Model file for the job. Use its own axes, mm. A direction names the side the tool comes from. Round coordinates to 2 decimals unless told otherwise and drop trailing zeros. Loops run counter-clockwise (first coordinate to the right, second up) from the corner with the lowest first, then second, coordinate; pieces in that order, holes last. Notation, with made-up numbers: (1, -32) -> (31, -32) arc R31 ccw to (31, 7) -> close; hole circle Ø1 at (75, -40). An arc over 180 degrees is marked (long way). Use a Markdown table: item, result. Add a question column.
```python
from build123d import *

# Parameters (mm, degrees)
EXTRUDE_1_DEPTH     = 4
CUT_EXTRUDE_1_DEPTH = 1.5
CUT_EXTRUDE_2_DEPTH = 7.5


with BuildPart() as part:
    # Эскиз1 → Бобышка-Вытянуть1 (new body, symmetric)
    with BuildSketch(Plane.XY):
        Polygon((4, 0), (-4, 0), (-4, -1.5), (-9.75, -1.5), (-9.75, -8), (9.75, -8), (9.75, -1.5), (4, -1.5), align=None)
    extrude(amount=EXTRUDE_1_DEPTH, both=True)

    # Эскиз3 → Отверстие обработанное метчиком M62 (revolve, cut)
    with BuildSketch(Plane(origin=(0, 0, 0), x_dir=(0, 0, 1), z_dir=(1, 0, 0))):
        Polygon((0, 0), (0, 8), (3.5, 8), (2.5, 7), (2.5, 1), (3.5, 0), align=None)
    revolve(axis=Axis((0, 6.35, 0), (0, -1, 0)), mode=Mode.SUBTRACT)

    # Эскиз4 → Вырез-Вытянуть1 (cut)
    with BuildSketch(Plane(origin=(0, 0, 0), x_dir=(1, 0, 0), z_dir=(0, 1, 0))):
        with BuildLine():
            Line((-4, 4), (-4, 0))
            ThreePointArc((-4, 0), (-2.828427125, 2.828427125), (0, 4))
            Line((0, 4), (-4, 4))
        make_face()
        with BuildLine():
            Line((0, -4), (4, -4))
            Line((4, -4), (4, 0))
            ThreePointArc((4, 0), (2.828427125, -2.828427125), (0, -4))
        make_face()
    extrude(amount=-CUT_EXTRUDE_1_DEPTH, mode=Mode.SUBTRACT)

    # Эскиз5 → Вырез-Вытянуть2 (cut, through all)
    with BuildSketch(Plane(origin=(0, -1.5, 0), x_dir=(1, 0, 0), z_dir=(0, 1, 0))):
        with BuildLine():
            Line((-9.75, 0), (-9.75, 4))
            Line((-9.75, 4), (-8.891709622, 4))
            ThreePointArc((-8.891709622, 4), (-9.533012871, 2.045523305), (-9.75, 0))
        make_face()
        with BuildLine():
            Line((9.75, 0), (9.75, -4))
            Line((9.75, -4), (8.891709622, -4))
            ThreePointArc((8.891709622, -4), (9.533012871, -2.045523305), (9.75, 0))
        make_face()
    extrude(amount=-CUT_EXTRUDE_2_DEPTH, mode=Mode.SUBTRACT)

    # Вырез-По траектории1: sweep along a path in Эскиз7
    with BuildLine(Plane.XZ.offset(8)) as sweep_1_path:
        Line((0, 9.75), (-9.75, 9.75))
        Line((-9.75, 9.75), (-9.75, 0))
        ThreePointArc((-9.75, 0), (-6.894291117, -6.894291117), (0, -9.75))
        Line((0, -9.75), (9.75, -9.75))
        Line((9.75, -9.75), (9.75, 0))
        ThreePointArc((9.75, 0), (6.894291117, 6.894291117), (0, 9.75))
    # Эскиз6 → Вырез-По траектории1 (sweep, cut)
    with BuildSketch(Plane.XY.offset(4)):
        Polygon((-9.75, -3), (-9.75, -8), (-4, -8), align=None)
    sweep(path=sweep_1_path.line, transition=Transition.RIGHT, mode=Mode.SUBTRACT)


solid = part.part
```
1) Cut at B-B on y = -6. Write the cut outline in (x, z).
2) Cut at A-A on y = -2. Write the cut outline in (x, z).
3) Wall check: probe 1 along Z at (x, y) = (0, -2.4); probe 2 along X at (y, z) = (-4, -1.5); probe 3 along X at (y, z) = (-5.3, 0) (3 decimals). Give the ranges that are in metal, low to high. Write a range as from..to.
4) Tool access for faces 1 (the face through (-2.859, -0.74, -2.797)), 2 (the face through (-4, -1, 2)), 3 (the face through (4, -1, -2)): list every direction of +Z, -Z, +X, -X, +Y, -Y with a clear straight run to the whole face (end or side of a thin tool).
5) Pin check, flat tips, straight feed: pin 1 Ø2.5 at (x, z) = (-6.5, 0) entering from +Y; pin 2 Ø1.6 at (y, z) = (-0.5, -2) entering from +X; pin 3 Ø1.2 at (y, z) = (-1, 3) entering from -X. Stop position of each tip, or through.
Established:
| question | item | result |
|---|---|---|
| 1 | outline | (-6.3, 0) arc R6.3 ccw to (-4.87, -4) -> (6.3, -4) -> (6.3, 0) arc R6.3 ccw to (4.87, 4) -> (-6.3, 4) -> close; hole circle Ø5 at (0, 0) |
| 2 | outline | (-9.75, 0) arc R9.75 ccw to (-8.89, -4) -> (9.75, -4) -> (9.75, 0) arc R9.75 ccw to (8.89, 4) -> (-9.75, 4) -> close; hole circle Ø5 at (0, 0) |
| 3 | probe 1 | z = -4..-2.5, 2.5..4 |
| 3 | probe 2 | x = -8.47..-2, 2..8.6 |
| 3 | probe 3 | x = -7.105..-2.5, 2.5..7.105 |
| 4 | face 1 | -Z, -X, +Y |
| 4 | face 2 | +Z, -Z, -X, +Y |
| 4 | face 3 | +Z, -Z, +X, +Y |
| 5 | pin 1 | stops at y = -1.5 |
| 5 | pin 2 | stops at x = 4 |
| 5 | pin 3 | stops at x = -9.75 |
